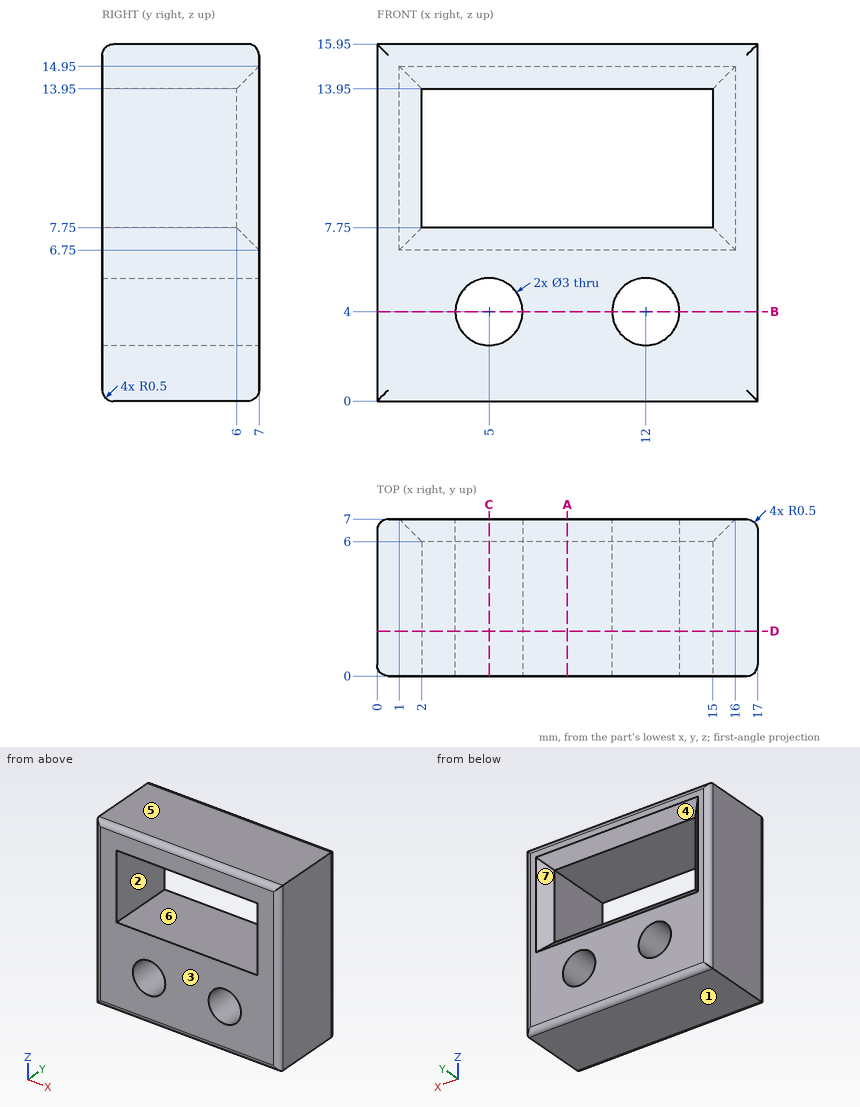
Study the drawing (mm; zero at the part's minimum x, y, z) and answer. A direction names the side the tool comes from. Round coordinates to 2 decimals unless told otherwise and drop trailing zeros. Write each loop counter-clockwise with the first axis right and the second up, starting at its lowest first coordinate (ties: lowest second). Pieces come first, ordered by that corner, then holes.
1) A tool of negligible diameter and unlimited length cuts with its end or side. For the marked faces 5, 6 and 7, from which of +Z, -Z, +X, -X, +Y, -Y can it reach the whole face along a straight path? Write none if from no direction.
2) A cutting plane is placed at D-D (y = 2). Give the vertices of the cut face in (x, z), plus the area to 3 significant figures.
3) Given pin 1 Ø1.5 at (x, z) = (7.5, 11.5) entering from -Y, flat-ended and moving along its own axis, determine where the tip first touches the part or whether it passes through.
4) The mould has two halves that part along Z. Classify the marked faces 1, 2, 3 and 4: pulls with the +Z half, pulls with the -Z half, needs draft (parallel to the pull), parting line crosses it, or undercut.
5) A cutting plane is placed at B-B (z = 4). Give the vertices of the cut face in (x, y).
6) A cutting plane is placed at A-A (x = 8.5). Give the vertices of the cut face in (y, z).
7) A cutting plane is placed at C-C (x = 5). Give the vertices of the cut face in (y, z), plus the area to 3 significant figures.
8) Straight lines are drawn through the part: line 1 (Z direction, x = 5, y = 4); line 2 (X direction, y = 3.25, z = 13); line 3 (Z direction, x = 13.75, y = 4.5). For each, find the intervals that lie inside material, in ascending order.
Completed:
1. face 5: +Z, +X, -X, +Y, -Y
1. face 6: +Y, -Y
1. face 7: +Y
2. outline: (0, 0) - (17, 0) - (17, 15.95) - (0, 15.95) - close; hole (2, 7.75) - (15, 7.75) - (15, 13.95) - (2, 13.95) - close; hole circle Ø3 at (5, 4); hole circle Ø3 at (12, 4)
2. area: 176 mm2
3. pin 1: passes through
4. face 1: pulls with the -Z half
4. face 2: undercut
4. face 3: needs draft
4. face 4: undercut
5. outline: (0, 0.5) arc R0.5 ccw to (0.5, 0) - (3.5, 0) - (3.5, 7) - (0.5, 7) arc R0.5 ccw to (0, 6.5) - close; (6.5, 0) - (10.5, 0) - (10.5, 7) - (6.5, 7) - close; (13.5, 0) - (16.5, 0) arc R0.5 ccw to (17, 0.5) - (17, 6.5) arc R0.5 ccw to (16.5, 7) - (13.5, 7) - close
6. outline: (0, 0.5) arc R0.5 ccw to (0.5, 0) - (6.5, 0) arc R0.5 ccw to (7, 0.5) - (7, 6.75) - (6, 7.75) - (0, 7.75) - close; (0, 13.95) - (6, 13.95) - (7, 14.95) - (7, 15.45) arc R0.5 ccw to (6.5, 15.95) - (0.5, 15.95) arc R0.5 ccw to (0, 15.45) - close
7. outline: (0, 0.5) arc R0.5 ccw to (0.5, 0) - (6.5, 0) arc R0.5 ccw to (7, 0.5) - (7, 2.5) - (0, 2.5) - close; (0, 5.5) - (7, 5.5) - (7, 6.75) - (6, 7.75) - (0, 7.75) - close; (0, 13.95) - (6, 13.95) - (7, 14.95) - (7, 15.45) arc R0.5 ccw to (6.5, 15.95) - (0.5, 15.95) arc R0.5 ccw to (0, 15.45) - close
7. area: 46.0 mm2
8. line 1: z = 0 to 2.5, 5.5 to 7.75, 13.95 to 15.95
8. line 2: x = 0 to 2, 15 to 17
8. line 3: z = 0 to 7.75, 13.95 to 15.95
